from build123d import *

# Parameters (mm, degrees)
F0_R     = 5
F1_ANGLE = 283.41057


with BuildPart() as f1:
    # F0 (on Top) → F1 (revolve)
    with BuildSketch(Plane.XY):
        Polygon((8.660254, -5), (8.660254, 5), (0, 10), (-8.660254, 5), (-8.660254, -5), (0, -10), align=None)
        Circle(F0_R, mode=Mode.SUBTRACT)
    revolve(axis=Axis((-36.425274, -12.058022, 0), (0, -1, 0)), revolution_arc=F1_ANGLE)


solid = f1.part
Model file for the job. Use its own axes, mm. A direction names the side the tool comes from. Give positions to 0.01 mm unless a question says otherwise; leave off trailing zeros. Order: outer loops, then holes, each group sorted by start corner. A loop starts at its lowest first (then second) coordinate and runs counter-clockwise, first axis right, second up. Notation, with made-up numbers: (82, 49) -> (129, 49) arc R19 cw to (129, 66) -> close; hole circle Ø9 at (-33, -35). An arc over 180 degrees is marked (long way). Use CSV: the item, a comma, the result in double quotes.
1. 3-axis set-ups, long thin cutter, end or side, ignore diameter. For faces 4 (the flat face through (-4, -4, 0)), 5 (the cylindrical face through (-57.61, -0.07, 17.95)): which of +Z, -Z, +X, -X, +Y, -Y reach the whole face in a straight line?
Outcome:
face 4,"-Z, +X, +Y, -Y"
face 5,"+Y, -Y"
2. Drop flat-ended pins along their axis: pin 1 (6 mm diameter, centred on y = 2, z = 19.5, fed in from -X); pin 2 (6 mm diameter, centred on x = -16, y = 1.5, fed in from +Z); pin 3 (8 mm diameter, centred on x = -12, y = -3.5, fed in from -Z). Give the stop position or say it passes through.
Outcome:
pin 1,"x = -78.38"
pin 2,"z = 41.58"
pin 3,"z = 0"
3. Drill centre lines: line 1 along Z through (x, y) = (-28, 4.5); line 2 along Z through (x, y) = (-43.5, -1.25); line 3 along Z through (x, y) = (-50.5, 2.5). Where is each one in solid material? Low to high. Write a range as from..to.
Outcome:
line 1,"-44.29..-37.67, 26.46..33.19, 37.67..44.29"
line 2,"-44.53..-40.66, -30.78..-26.85, 26.85..30.78, 40.66..44.53"
line 3,"-42.83..-38.25, -28.84..-23.93, 23.93..28.84, 38.25..42.83"
4. Band-saw the part on A-A, the plane y = 3.5. Give the cut face in (x, z), then the cut area to 3 significant figures.
Outcome:
outline,"(-29.99, -27.01) arc R27.77 cw (long way) to (-8.66, 0) -> (-3.57, 0) arc R32.85 ccw (long way) to (-28.81, -31.96) -> close; (-27.15, -38.91) arc R40 cw (long way) to (3.57, 0) -> (8.66, 0) arc R45.09 ccw (long way) to (-25.97, -43.86) -> close"
area,"1,830 mm²"
5. Band-saw the part on B-B, the plane x = -53. Count the separate pieces of the cut face and the enclosed holes in it, then the cut area to 3 significant figures.
Outcome:
separate pieces,"2"
enclosed holes,"2"
area,"412 mm²"
6. Mould opens along X. For faces 1 (the flat face through (-28.9, -4.3, -31.57)), 2 (the conical face through (-58.02, -5.31, 18.3)), 3 (the conical face through (-64.535, 9.757, 23.821)) say: +X half, -X half, draft (parallel to the pull), parting line (faces both ways), or undercut.
Outcome:
face 1,"+X half"
face 2,"undercut"
face 3,"parting line"
